For this review, take the finished solid that the model builds, in its own axes (mm). A direction names the side the tool comes from. Round coordinates to 2 decimals unless told otherwise and drop trailing zeros. Write each loop counter-clockwise with the first axis right and the second up, starting at its lowest first coordinate (ties: lowest second). Pieces come first, ordered by that corner, then holes. Notation, with made-up numbers: (56, 75) -> (75, 75) arc R19 ccw to (75, 85) -> close; hole circle Ø7 at (-3.75, 85). An arc over 180 degrees is marked (long way). Answer in a Markdown table with one row per item.
from build123d import *

# Parameters (mm, degrees)
EXTRUDE_1_DEPTH = 35
EXTRUDE_2_DEPTH = 2


with BuildPart() as part:
    # 草图1 → 凸台-拉伸1 (new body)
    with BuildSketch(Plane(origin=(0, 0, 0), x_dir=(0, 0, -1), z_dir=(1, 0, 0))):
        Polygon((-44, 0), (44, 0), (44, 6), (19, 6), (19, 26), (15, 26), (15, 6), (-15, 6), (-15, 26), (-19, 26), (-19, 6), (-44, 6), align=None)
    extrude(amount=EXTRUDE_1_DEPTH)

    # 草图2 → 凸台-拉伸2 (add)
    with BuildSketch(Plane.XZ):
        with BuildLine():
            Line((35, 27.213074887), (35, 32.682458366))
            ThreePointArc((35, 32.682458366), (17.5, 43), (0, 32.682458366))
            Line((0, 32.682458366), (0, 27.213074887))
            ThreePointArc((0, 27.213074887), (17.5, 41), (35, 27.213074887))
        make_face()
        with BuildLine():
            Line((35, 13.317541634), (35, 18.786925113))
            ThreePointArc((35, 18.786925113), (17.5, 5), (0, 18.786925113))
            Line((0, 18.786925113), (0, 13.317541634))
            ThreePointArc((0, 13.317541634), (17.5, 3), (35, 13.317541634))
        make_face()
        with BuildLine():
            Line((35, -18.786925113), (35, -13.317541634))
            ThreePointArc((35, -13.317541634), (17.5, -3), (0, -13.317541634))
            Line((0, -13.317541634), (0, -18.786925113))
            ThreePointArc((0, -18.786925113), (17.5, -5), (35, -18.786925113))
        make_face()
        with BuildLine():
            Line((0, -27.213074887), (0, -32.682458366))
            ThreePointArc((0, -32.682458366), (17.5, -43), (35, -32.682458366))
            Line((35, -32.682458366), (35, -27.213074887))
            ThreePointArc((35, -27.213074887), (17.5, -41), (0, -27.213074887))
        make_face()
    extrude(amount=EXTRUDE_2_DEPTH)


solid = part.part
1) Consider section D-D on x = 11.5. State the section outline as (y, z) points, then the cut area to 3 significant figures.
Solved:
| item | result |
|---|---|
| outline | (-2, -42.08) -> (0, -42.08) -> (0, -44) -> (6, -44) -> (6, -19) -> (26, -19) -> (26, -15) -> (6, -15) -> (6, 15) -> (26, 15) -> (26, 19) -> (6, 19) -> (6, 44) -> (0, 44) -> (0, 42.08) -> (-2, 42.08) -> (-2, 39.97) -> (0, 39.97) -> (0, 6.03) -> (-2, 6.03) -> (-2, 3.92) -> (0, 3.92) -> (0, -3.92) -> (-2, -3.92) -> (-2, -6.03) -> (0, -6.03) -> (0, -39.97) -> (-2, -39.97) -> close |
| area | 705 mm² |
2) Mouldability with a two-part tool opening along Z and no side actions: class faces 6 (the cylindrical face through (17.202, -0.986, -42.998)), 7 (the flat face through (17, 0, 23)), 8 (the cylindrical face through (17.164, -0.986, -5.003)), 9 (the flat face through (17, 6, 31)) as pulls with the +Z half, pulls with the -Z half, needs draft (parallel to the pull), parting line crosses it, or undercut.
Solved:
| item | result |
|---|---|
| face 6 | pulls with the -Z half |
| face 7 | undercut |
| face 8 | undercut |
| face 9 | needs draft |
3) Clearance check with flat-ended pins moving along their axes: pin 1 Ø12.5 at (x, z) = (25.5, -35.5) entering from +Y; pin 2 Ø17.5 at (x, z) = (22, 29.5) entering from -Y; pin 3 Ø1.5 at (x, y) = (14.5, 15.5) entering from -Z. State where each tip first meets the part, or that it passes through.
Solved:
| item | result |
|---|---|
| pin 1 | y = 6 |
| pin 2 | y = 0 |
| pin 3 | z = -19 |
4) Consider section C-C on z = -29. State the section outline as (x, y) points.
Solved:
| item | result |
|---|---|
| outline | (0, -2) -> (0.53, -2) -> (0.53, 0) -> (34.47, 0) -> (34.47, -2) -> (35, -2) -> (35, 6) -> (0, 6) -> close |
5) Consider section B-B on x = 25. State the section outline as (y, z) points.
Solved:
| item | result |
|---|---|
| outline | (-2, -41.54) -> (0, -41.54) -> (0, -44) -> (6, -44) -> (6, -19) -> (26, -19) -> (26, -15) -> (6, -15) -> (6, 15) -> (26, 15) -> (26, 19) -> (6, 19) -> (6, 44) -> (0, 44) -> (0, 41.54) -> (-2, 41.54) -> (-2, 39.36) -> (0, 39.36) -> (0, 6.64) -> (-2, 6.64) -> (-2, 4.46) -> (0, 4.46) -> (0, -4.46) -> (-2, -4.46) -> (-2, -6.64) -> (0, -6.64) -> (0, -39.36) -> (-2, -39.36) -> close |
6) For faces 1 (the cylindrical face through (17.164, -0.986, 40.997)), 2 (the flat face through (17, 16, -15)), 3 (the flat face through (17, 16, 19)), 4 (the cylindrical face through (17.798, -0.986, 42.998)), 5 (the flat face through (17, 6, -32)), list the 3-axis set-ups (+Z, -Z, +X, -X, +Y, -Y) from which the entire face can be reached by the end or side of a thin tool; tool diameter is ignored.
Solved:
| item | result |
|---|---|
| face 1 | -Y |
| face 2 | +X, -X, +Y |
| face 3 | +Z, +X, -X, +Y |
| face 4 | +Z, -Y |
| face 5 | -Z, +X, -X, +Y |
7) For line 1 (Z direction, x = 24.5, y = 7.25); line 2 (Y direction, x = 32.5, z = 10.5); line 3 (Y direction, x = 7.5, z = -29.5), list the stretches that pass through material, from the lowest coordinate up. Write a range as [from, to].
Solved:
| item | result |
|---|---|
| line 1 | [-19, -15], [15, 19] |
| line 2 | [-2, 6] |
| line 3 | [0, 6] |
8) Consider section A-A on y = 18.5. State the section outline as (x, z) points, then the cut area to 3 significant figures.
Solved:
| item | result |
|---|---|
| outline | (0, -19) -> (35, -19) -> (35, -15) -> (0, -15) -> close; (0, 15) -> (35, 15) -> (35, 19) -> (0, 19) -> close |
| area | 280 mm² |
